from build123d import *

# Parameters (mm, degrees)
IZIM1_W                     = 80
IZIM1_H                     = 80
IZIM1_R                     = 2.5
Y_KSEKLIK_EKSTR_ZYON1_DEPTH = 20
KES_EKSTR_ZYON2_DEPTH       = 61
KES_EKSTR_ZYON3_START       = 10
KES_EKSTR_ZYON3_DEPTH       = 10
M4X0_7_DI_LI_DELIK1_D       = 3.3


# Read off the part's stored shape, not the designer's step: Kes-Ekstrüzyon3
with BuildPart() as part:
    # Çizim1 → Yükseklik-Ekstrüzyon1 (new body)
    with BuildSketch(Plane(origin=(0, 0, 0), x_dir=(1, 0, 0), z_dir=(0, 1, 0))):
        Rectangle(IZIM1_W, IZIM1_H)
        with Locations(Location((-30, 30, 0), (0, 0, 270))):
            Circle(IZIM1_R, mode=Mode.SUBTRACT)
        with Locations(Location((30, 30, 0), (0, 0, 270))):
            Circle(IZIM1_R, mode=Mode.SUBTRACT)
        with Locations(Location((-30, -30, 0), (0, 0, 270))):
            Circle(IZIM1_R, mode=Mode.SUBTRACT)
        with Locations(Location((30, -30, 0), (0, 0, 270))):
            Circle(IZIM1_R, mode=Mode.SUBTRACT)
    extrude(amount=Y_KSEKLIK_EKSTR_ZYON1_DEPTH)

    # Çizim2 → Kes-Ekstrüzyon2 (cut, through all)
    with BuildSketch(Plane(origin=(0, 20, 0), x_dir=(1, 0, 0), z_dir=(0, 1, 0))):
        with BuildLine():
            Line((-10, 8.426169555), (-10, -7.573830445))
            ThreePointArc((-10, -7.573830445), (-15, -12.573830445), (-20, -7.573830445))
            Line((-20, -7.573830445), (-20, 8.426169555))
            ThreePointArc((-20, 8.426169555), (-15, 13.426169555), (-10, 8.426169555))
        make_face()
        with BuildLine():
            Line((20, 8), (20, -8))
            ThreePointArc((20, -8), (15, -13), (10, -8))
            Line((10, -8), (10, 8))
            ThreePointArc((10, 8), (15, 13), (20, 8))
        make_face()
    extrude(amount=-KES_EKSTR_ZYON2_DEPTH, mode=Mode.SUBTRACT)

    # Kes-Ekstrüzyon3 outline → Kes-Ekstrüzyon3 (cut)
    # profile 1 of 2: a face of its own
    with BuildSketch(Plane(origin=(0, 0, 0), x_dir=(1, 0, 0), z_dir=(0, 1, 0)).offset(KES_EKSTR_ZYON3_START)):
        with BuildLine():
            Line((-25, 8.426169555), (-25, -7.573830445))
            ThreePointArc((-25, -7.573830445), (-15, -17.573830445), (-5, -7.573830445))
            Line((-5, -7.573830445), (-5, 8.426169555))
            ThreePointArc((-5, 8.426169555), (-15, 18.426169555), (-25, 8.426169555))
        make_face()
        with BuildLine():
            ThreePointArc((-20, 8.426169555), (-15, 13.426169555), (-10, 8.426169555))
            Line((-10, 8.426169555), (-10, -7.573830445))
            ThreePointArc((-10, -7.573830445), (-15, -12.573830445), (-20, -7.573830445))
            Line((-20, -7.573830445), (-20, 8.426169555))
        make_face(mode=Mode.SUBTRACT)
    # profile 2 of 2: a face of its own
    with BuildSketch(Plane(origin=(0, 0, 0), x_dir=(1, 0, 0), z_dir=(0, 1, 0)).offset(KES_EKSTR_ZYON3_START)):
        with BuildLine():
            Line((25, -8), (25, 8))
            ThreePointArc((25, 8), (15, 18), (5, 8))
            Line((5, 8), (5, -8))
            ThreePointArc((5, -8), (15, -18), (25, -8))
        make_face()
        with BuildLine():
            ThreePointArc((10, 8), (15, 13), (20, 8))
            Line((20, 8), (20, -8))
            ThreePointArc((20, -8), (15, -13), (10, -8))
            Line((10, -8), (10, 8))
        make_face(mode=Mode.SUBTRACT)
    extrude(amount=KES_EKSTR_ZYON3_DEPTH, mode=Mode.SUBTRACT)

    # M4x0.7 Dişli Delik1 (through all)
    with Locations(Plane(origin=(0, 20, 0), x_dir=(1, 0, 0), z_dir=(0, 1, 0))):
        with Locations((0, 19.118083018)):
            Hole(M4X0_7_DI_LI_DELIK1_D / 2)


solid = part.part
Verification items for the finished model (mm, model axes). A direction names the side the tool comes from. Give positions to 0.01 mm unless a question says otherwise; leave off trailing zeros. Loops run counter-clockwise (first coordinate to the right, second up) from the corner with the lowest first, then second, coordinate; pieces in that order, holes last. Notation, with made-up numbers: (-2.5, 2) - (11.5, 2) arc R19 ccw to (11.5, 32) - close; hole circle Ø11 at (46, 36). An arc over 180 degrees is marked (long way). Write item = value, one per line. Start each with the question number.
Q1. Thickness scan on line 1 (X direction, y = 8.5, z = -30); line 2 (Z direction, x = 0, y = 6.25); line 3 (Z direction, x = -11.5, y = 1). Record the ranges inside material, lowest first.
Q2. Cross-section at C-C, the plane x = -30. Enter the section's corners in (y, z), and give its area (3 significant figures).
Q3. Tool access check on faces 4 (the face through (-20, 5, 0)), 5 (the face through (-14.78, 14.93, -18.424)), 6 (the face through (-1, 20, -1)). Record the directions out of +Z, -Z, +X, -X, +Y, -Y that give a thin tool (end or side, any length) a straight path to the whole face; none if there is none.
Q4. Depth check by flat-ended pin: P1, Ø4, axis at x = -30, z = 30, coming from the -Y side; P2, Ø10, axis at x = -19, z = 2.5, coming from the +Y side. Enter the tip coordinate at first touch or a pass-through.
Q5. Cross-section at A-A, the plane z = -30. Enter the section's corners in (x, y), and give its area (3 significant figures).
Q6. Cross-section at B-B, the plane x = -15. Enter the section's corners in (y, z).
Q7. Cross-section at D-D, the plane z = 1.5. Enter the section's corners in (x, y).
Q8. Mould release check, pull along X, two halves, no side actions. Record for faces 1 (the face through (-1, 10, 40)), 2 (the face through (40, 10, 1)), 3 (the face through (20, 5, 0)): released by +X, released by -X, zero draft, split by the parting line, or undercut.
Answer key:
q1.line_1 = -40 to -32.5, -27.5 to 27.5, 32.5 to 40
q1.line_2 = -40 to -20.77, -17.47 to 40
q1.line_3 = -40 to -12, 11.14 to 40
q2.outline = (0, -40) - (20, -40) - (20, -32.5) - (0, -32.5) - close; (0, -27.5) - (20, -27.5) - (20, 27.5) - (0, 27.5) - close; (0, 32.5) - (20, 32.5) - (20, 40) - (0, 40) - close
q2.area = 1,400 mm^2
q3.face_4 = +Y, -Y
q3.face_5 = +Y
q3.face_6 = +Z, -Z, +X, -X, +Y
q4.P1 = through
q4.P2 = 10
q5.outline = (-40, 0) - (-32.5, 0) - (-32.5, 20) - (-40, 20) - close; (-27.5, 0) - (27.5, 0) - (27.5, 20) - (-27.5, 20) - close; (32.5, 0) - (40, 0) - (40, 20) - (32.5, 20) - close
q5.area = 1,400 mm^2
q6.outline = (0, -40) - (20, -40) - (20, -18.43) - (10, -18.43) - (10, -13.43) - (0, -13.43) - close; (0, 12.57) - (10, 12.57) - (10, 17.57) - (20, 17.57) - (20, 40) - (0, 40) - close
q7.outline = (-40, 0) - (-20, 0) - (-20, 10) - (-25, 10) - (-25, 20) - (-40, 20) - close; (-10, 0) - (10, 0) - (10, 10) - (5, 10) - (5, 20) - (-5, 20) - (-5, 10) - (-10, 10) - close; (20, 0) - (40, 0) - (40, 20) - (25, 20) - (25, 10) - (20, 10) - close
q8.face_1 = zero draft
q8.face_2 = released by +X
q8.face_3 = undercut
